Answer from the drawing. Dimensions are ordinates in mm from the lowest x, y and z of the part. A direction names the side the tool comes from. Give positions to 0.01 mm unless a question says otherwise; leave off trailing zeros. Order: outer loops, then holes, each group sorted by start corner. A loop starts at its lowest first (then second) coordinate and runs counter-clockwise, first axis right, second up. Notation, with made-up numbers: (2.5, 55) -> (7.5, 55) arc R14 cw to (7.5, 79) -> close; hole circle Ø7 at (8.25, 77). An arc over 180 degrees is marked (long way). Answer as CSV lines item,"result". Start each with the question number.
1) The mould has two halves that part along Z. Classify the marked faces 1, 2, 3 and 4: +Z half, -Z half, draft (parallel to the pull), parting line (faces both ways), or undercut.
2) Flat-ended cylindrical pins translate along their axes: pin 1 Ø10 at (y, z) = (91, 35.5) entering from +X; pin 2 Ø16 at (y, z) = (68, 11) entering from -X; pin 3 Ø6 at (y, z) = (64.5, 7.5) entering from +X. Find the tip coordinate at first contact, or state that the pin passes through.
3) Find section A-A (x = 108.5). Determine the outline of the cut face in (y, z), and give its area (3 significant figures).
4) Find section B-B (y = 30.5). Determine the outline of the cut face in (x, z).
5) Find section C-C (z = 34.5). Determine the outline of the cut face in (x, y), and give its area (3 significant figures).
6) Straight lines are drawn through the part: L1, parallel to Z at x = 17.5, y = 28; L2, parallel to X at y = 110, z = 68; L3, parallel to X at y = 22, z = 7. For each, find the intervals that lie inside material, in ascending order. Write a range as from..to.
7) For the marked faces 5, 6 and 7, determine the directions among +Z, -Z, +X, -X, +Y, -Y from which every point of the face is accessible in a straight line to the end or side of a thin tool.
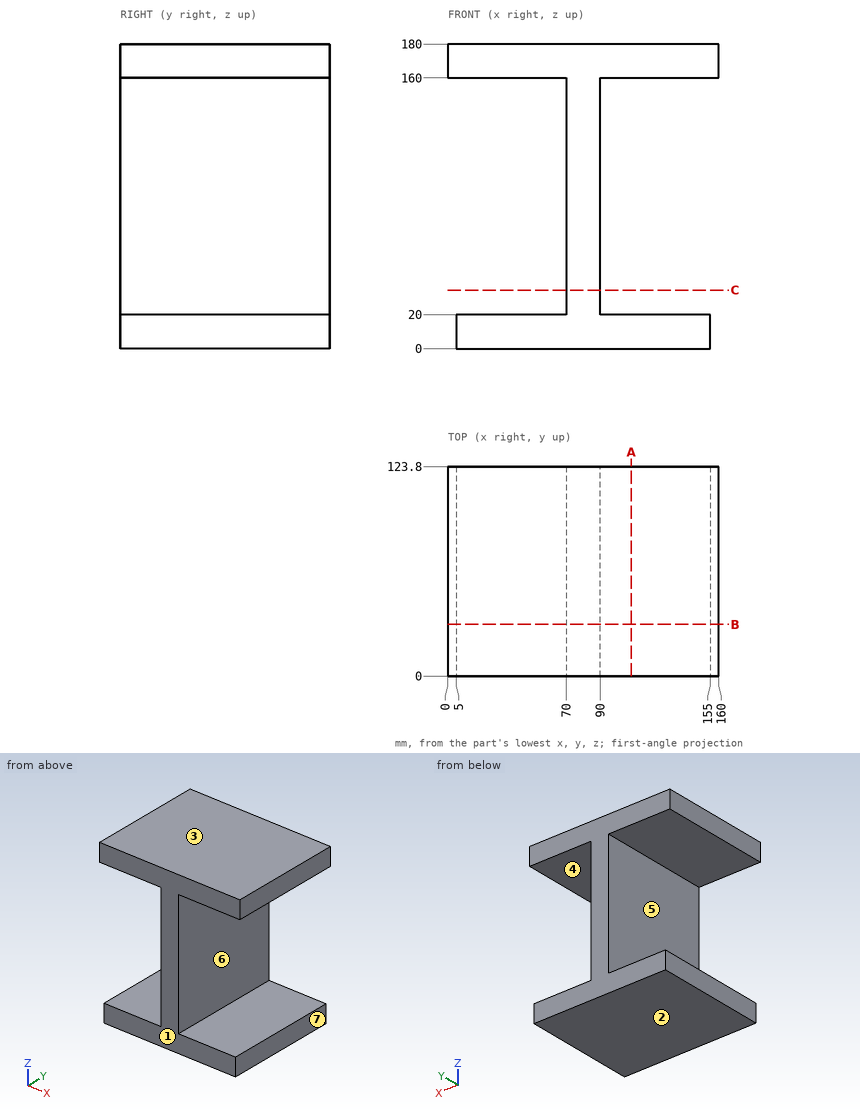
Findings below:
1,face 1,"draft"
1,face 2,"-Z half"
1,face 3,"+Z half"
1,face 4,"undercut"
2,pin 1,"x = 90"
2,pin 2,"x = 5"
2,pin 3,"x = 155"
3,outline,"(0, 0) -> (123.8, 0) -> (123.8, 20) -> (0, 20) -> close; (0, 160) -> (123.8, 160) -> (123.8, 180) -> (0, 180) -> close"
3,area,"4,950 mm²"
4,outline,"(0, 160) -> (70, 160) -> (70, 20) -> (5, 20) -> (5, 0) -> (155, 0) -> (155, 20) -> (90, 20) -> (90, 160) -> (160, 160) -> (160, 180) -> (0, 180) -> close"
5,outline,"(70, 0) -> (90, 0) -> (90, 123.8) -> (70, 123.8) -> close"
5,area,"2,480 mm²"
6,L1,"0..20, 160..180"
6,L2,"70..90"
6,L3,"5..155"
7,face 5,"-X, +Y, -Y"
7,face 6,"+X, +Y, -Y"
7,face 7,"-Z, +X, +Y, -Y"
